Autodesk Fusion 360 part; units mm, degrees
sketch "Skizze1" plane through (0, 0, 0) normal (0, 0, 1) x (1, 0, 0)
  line L0 (0, 0) -> (0, 25)
  line L1 (0, 0) -> (20, 0)
  line L2 (0, 25) -> (3, 25)
  line L3 (17, 3) -> (9, 3)
  line L4 (3, 25) -> (9, 3)
  line L5 (3, 25) -> (3, 3) construction
  line L6 (3, 3) -> (9, 3) construction
  line L7 (17, 6) -> (20, 0)
  line L8 (17, 6) -> (16.1818, 6)
  line L9 (17, 3) -> (16.1818, 6)
  line L10 (17, 3) -> (22, 3) construction
  dimension "d1" = 3
  dimension "d4" = 74.745
  dimension "d5" = 105.255
extrude "Extrusion1" add sketch "Skizze1" along normal blind 10
sketch "Skizze3" plane through (0, 0, 0) normal (0, 0, -1) x (1, 0, 0)
  line L0 (20, 0) -> (0, 0)
  line L1 (0, 0) -> (0, -25)
  line L2 (0, -25) -> (3, -25)
  line L3 (3, -25) -> (9, -3)
  line L4 (9, -3) -> (17, -3)
  line L5 (17, -3) -> (16.1818, -6)
  line L6 (16.1818, -6) -> (17, -6)
  line L7 (17, -6) -> (20, 0)
  line L8 (17, -3) -> (18.5, -3)
  line L9 (18.5, -3) -> (17, -6) construction
sketch "Skizze4" plane through (16, 8, 0) normal (0.8944, 0.4472, 0) x (-0.4472, 0.8944, 0)
  line L0 (-8.9443, 0) -> (-2.2361, 0)
  line L1 (-2.2361, 0) -> (-2.2361, 10)
  line L2 (-2.2361, 10) -> (-8.9443, 10)
  line L3 (-8.9443, 10) -> (-8.9443, 0)
  line L4 (-8.9443, 10) -> (-8.9443, 0) construction
  line L5 (-8.9443, 5) -> (-2.2361, 5) construction
  line L6 (-8.9443, 2.5) -> (-2.2361, 2.5) construction
  line L7 (-8.9443, 7.5) -> (-2.2361, 7.5) construction
  line L8 (-2.2361, 7.5) -> (-8.9443, 5)
  line L9 (-2.2361, 2.5) -> (-8.9443, 5)
  line L10 (-2.2361, 0) -> (-5.5902, 0) construction
  line L11 (-5.5902, 0) -> (-5.5902, 10) construction
  line L12 (-5.5902, 3.75) -> (-5.5902, 6.25)
  dimension "d10" = 2.5
  dimension "d11" = 2.5
  dimension "d13" = 3.3541
  dimension "d14" = 6.7082
extrude "Extrusion2" cut sketch "Skizze4" against normal blind 1.5 contours L1 L8 L9 L12
extrude "Extrusion3" cut 1 faces at (16.52, 5.76, 5.8333) along direction (-0.447214, 0.894427, 0) blind 0.4
extrude "Extrusion4" add 1 faces at (16.9348, 2.7764, 4.5833) along direction (0.894427, 0.447214, 0) blind 1.5
equation "d5 = 180 deg - 74.7448809423 deg"
properties part number "Konfiguration 1"
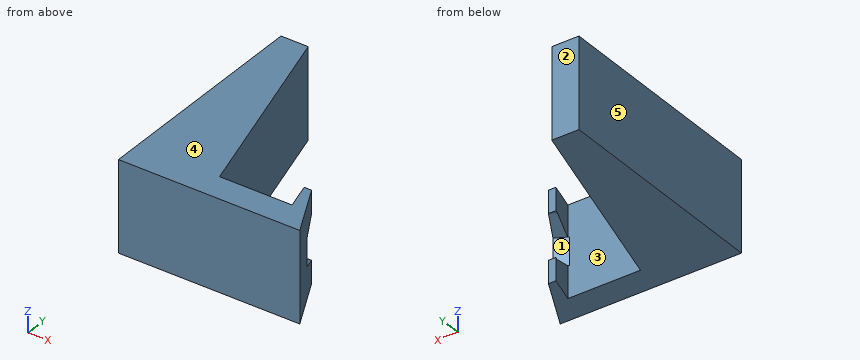
Build history of the part. All positions in model axes, mm. Face numbers are marked on the shaded views. A direction names the side the tool comes from. Give positions to 0.01 mm unless a question says otherwise; leave off trailing zeros. Order: outer loops, then holes, each group sorted by start corner. A loop starts at its lowest first (then second) coordinate and runs counter-clockwise, first axis right, second up. Notation, with made-up numbers: M 37,-12.75 L 90,-12.75 A16 ccw 90,8.25 Z; hole C 61,68 d10. An arc over 180 degrees is marked long. Write item = value, one per line. Start each with the question number.
(1) Slice it at C-C on y = 22.25. Write the cut outline in (x, z).
(2) Probe L1, parallel to Y at x = 14.75, z = 8.75; L2, parallel to X at y = 1.5, z = 0.5; L3, parallel to X at y = 9, z = 1. List the from-to ranges inside material, lowest first. Write a range as [from, to].
(3) Slice it at D-D on z = 0.75. Write the cut outline in (x, y), plus the area to 3 significant figures.
(4) Two-plate mould, pull along X, no slides. Class the marked faces 3, 4 and 5: released by +X, released by -X, zero draft, split by the parting line, or undercut.
(5) Pin check, flat tip, straight feed: pin 1 Ø0.7 at (x, z) = (16.5, 1.5) entering from +Y. Stop position of the tip, or through.
(6) Which spindle directions (+Z, -Z, +X, -X, +Y, -Y) get a long thin tool onto all of the face, cutting with end or side? Do the marked faces 1 and 2. Say none if no direction does.
(7) Slice it at B-B on x = 11.5. Write the cut outline in (y, z), plus the area to 3 significant figures.
(8) Slice it at A-A on z = 5.25. Write the cut outline in (x, y).
Responses:
q1.outline = M 0,0 L 3.75,0 L 3.75,10 L 0,10 Z
q2.L1 = [0, 3]
q2.L2 = [0, 19.25]
q2.L3 = [0, 7.36]
q3.outline = M 0,0 L 20,0 L 17,6 L 16.18,6 L 17,3 L 9,3 L 3,25 L 0,25 Z
q3.area = 193 mm2
q4.face_3 = undercut
q4.face_4 = zero draft
q4.face_5 = released by -X
q5.pin_1 = 6
q6.face_1 = +Y
q6.face_2 = +Z, -Z, +X, -X, +Y
q7.outline = M 0,0 L 3,0 L 3,10 L 0,10 Z
q7.area = 30.0 mm2
q8.outline = M 0,0 L 20,0 L 18.16,3.67 L 16.82,3 L 9,3 L 3,25 L 0,25 Z
